Read the model definition and answer for the solid it produces. Units are mm, in the model's axes. Face numbers are marked on the shaded views. A direction names the side the tool comes from. Coordinates: 2 decimals unless noted, no trailing zeros. Order: outer loops, then holes, each group sorted by start corner. A loop starts at its lowest first (then second) coordinate and runs counter-clockwise, first axis right, second up. Notation, with made-up numbers: M 8.5,1.25 L 14.5,1.25 A10 ccw 14.5,7.25 Z; hole C 23.5,85.25 d6. An arc over 180 degrees is marked long. One line per question, with ' | ' between items. Start each with the question number.
1) Consider probe 1 along Y at (x, z) = (29, 6.5); probe 2 along Z at (x, y) = (29, -26.5); probe 3 along X at (y, z) = (-28, 14). Determine where each line is inside the solid, lowest interval first.
2) Given P1, Ø3, axis at x = 15, z = 5, coming from the -Y side; P2, Ø6, axis at y = -30.5, z = 37.5, coming from the -X side, each flat-ended and moving along its own axis, determine where each tip first touches the part or whether it passes through.
3) Find section B-B, the plane x = 33. Write down the section's boundary in (y, z), plus the area to 3 significant figures.
4) A tool of negligible diameter and unlimited length cuts with its end or side. For the marked faces 1 and 2, from which of +Z, -Z, +X, -X, +Y, -Y can it reach the whole face along a straight path? Write none if from no direction.
5) Find section C-C, the plane y = -20. Write down the section's boundary in (x, z), plus the area to 3 significant figures.
6) The mould has two halves that part along Z. Classify the marked faces 3, 4 and 5: +Z half, -Z half, draft (parallel to the pull), parting line (faces both ways), or undercut.
7) Find section D-D, the plane z = 33.5. Write down the section's boundary in (x, y), plus the area to 3 significant figures.
8) Find section A-A, the plane z = 17. Write down the section's boundary in (x, y) (3 decimals).
from build123d import *

# Parameters (mm, degrees)
F0_W     = 57.522915
F0_H     = 45.961969
F0_R     = 13.727632
F1_DEPTH = 25.4
F2_DEPTH = 25.4
F0_R_2   = 10.083069
F3_DEPTH = 42.418


with BuildPart() as f1:
    # F0 (on Front) → F1 (new body)
    with BuildSketch(Plane.XZ):
        with Locations((28.761457, 22.980984)):
            Rectangle(F0_W, F0_H)
        with Locations((29.250471, 22.477599)):
            Circle(F0_R, mode=Mode.SUBTRACT)
    extrude(amount=F1_DEPTH)

    # F0 (on Front) → F2 (join)
    with BuildSketch(Plane.XZ):
        with Locations((28.761457, 22.980984)):
            Rectangle(F0_W, F0_H)
        with Locations((29.250471, 22.477599)):
            Circle(F0_R, mode=Mode.SUBTRACT)
    extrude(amount=F2_DEPTH)

    # F0 (on Front) → F3 (join)
    with BuildSketch(Plane.XZ):
        with Locations((29.250471, 22.477599)):
            Circle(F0_R)
        with Locations((29.250471, 22.477599)):
            Circle(F0_R_2, mode=Mode.SUBTRACT)
    extrude(amount=F3_DEPTH)


solid = f1.part
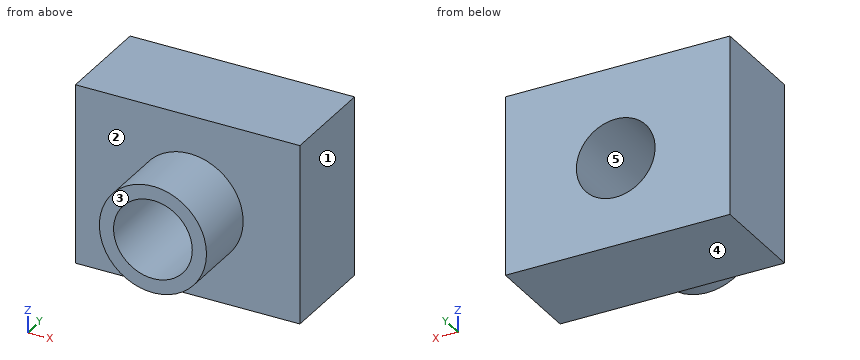
Report:
1) probe 1: y = -25.4 to 0 | probe 2: z = 8.75 to 12.4, 32.56 to 36.2 | probe 3: x = 18.45 to 23.79, 34.71 to 40.05
2) P1: stops at y = -25.4 | P2: stops at x = 22.62
3) outline: M -42.42,9.27 L -25.4,9.27 L -25.4,0 L 0,0 L 0,13.12 L -42.42,13.12 Z; M -42.42,31.84 L 0,31.84 L 0,45.96 L -25.4,45.96 L -25.4,35.68 L -42.42,35.68 Z | area: 823 mm^2
4) face 1: +Z, -Z, +X, +Y, -Y | face 2: -Y
5) outline: M 0,0 L 57.52,0 L 57.52,45.96 L 0,45.96 Z; hole C 29.25,22.48 d20.17 | area: 2,320 mm^2
6) face 3: draft | face 4: -Z half | face 5: undercut
7) outline: M 0,-25.4 L 21.07,-25.4 L 21.07,-42.42 L 37.43,-42.42 L 37.43,-25.4 L 57.52,-25.4 L 57.52,0 L 0,0 Z | area: 1,740 mm^2
8) outline: M 0,-25.4 L 16.663,-25.4 L 16.663,-42.418 L 20.785,-42.418 L 20.785,0 L 0,0 Z; M 37.716,-42.418 L 41.838,-42.418 L 41.838,-25.4 L 57.523,-25.4 L 57.523,0 L 37.716,0 Z
